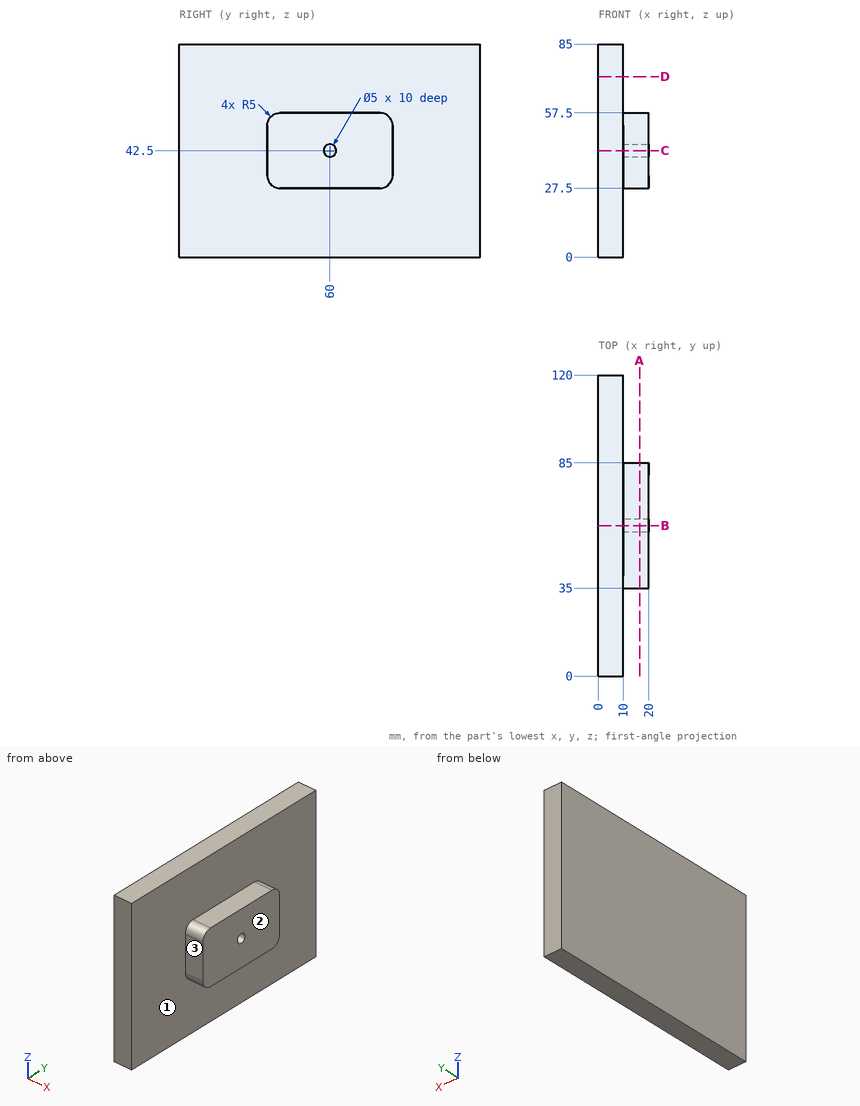
Geometry: see drawing. Coordinates: mm, zero at the bounding-box minimum. A direction names the side the tool comes from. Round coordinates to 2 decimals unless told otherwise and drop trailing zeros. Loops run counter-clockwise (first coordinate to the right, second up) from the corner with the lowest first, then second, coordinate; pieces in that order, holes last. Notation, with made-up numbers: (3, -5.75) -> (53, -5.75) arc R9 ccw to (53, 1.25) -> close; hole circle Ø6 at (-29.5, 2). An arc over 180 degrees is marked (long way). One line per question, with ' | ' between items. Start each with the question number.
1. Section B-B on y = 60. Output: boundary loops of the cut face in (x, z), and give its area (3 significant figures).
2. Line query: line 1 along Z through (x, y) = (16, 60); line 2 along X through (y, z) = (42.5, 62); line 3 along Y through (x, z) = (16, 35). Output: solid intervals per line, ascending. Write a range as [from, to].
3. Section D-D on z = 72. Output: boundary loops of the cut face in (x, y), and give its area (3 significant figures).
4. Section C-C on z = 42.5. Output: boundary loops of the cut face in (x, y), and give its area (3 significant figures).
5. Section A-A on x = 16.5. Output: boundary loops of the cut face in (y, z), and give its area (3 significant figures).
6. Contact query for flat-ended pins moving along their axis: pin 1 (5 mm diameter, centred on x = 16, z = 46.5, fed in from -Y); pin 2 (3 mm diameter, centred on x = 13, y = 50, fed in from +Z); pin 3 (5 mm diameter, centred on x = 13, z = 38, fed in from +Y). Output: stop coordinate, or through.
7. Set-up query: the marked faces 1, 2 and 3. Return all of +Z, -Z, +X, -X, +Y, -Y with unobstructed straight access to the full face (end or side cutting, diameter ignored); none if empty.
Returned:
1) outline: (0, 0) -> (10, 0) -> (10, 27.5) -> (20, 27.5) -> (20, 40) -> (10, 40) -> (10, 45) -> (20, 45) -> (20, 57.5) -> (10, 57.5) -> (10, 85) -> (0, 85) -> close | area: 1,100 mm2
2) line 1: z = [27.5, 40], [45, 57.5] | line 2: x = [0, 10] | line 3: y = [35, 85]
3) outline: (0, 0) -> (10, 0) -> (10, 120) -> (0, 120) -> close | area: 1,200 mm2
4) outline: (0, 0) -> (10, 0) -> (10, 35) -> (20, 35) -> (20, 57.5) -> (10, 57.5) -> (10, 62.5) -> (20, 62.5) -> (20, 85) -> (10, 85) -> (10, 120) -> (0, 120) -> close | area: 1,650 mm2
5) outline: (35, 32.5) arc R5 ccw to (40, 27.5) -> (80, 27.5) arc R5 ccw to (85, 32.5) -> (85, 52.5) arc R5 ccw to (80, 57.5) -> (40, 57.5) arc R5 ccw to (35, 52.5) -> close; hole circle Ø5 at (60, 42.5) | area: 1,460 mm2
6) pin 1: stops at y = 35 | pin 2: stops at z = 57.5 | pin 3: stops at y = 85
7) face 1: +X | face 2: +Z, -Z, +X, +Y, -Y | face 3: +Z, -Z, +X, -Y
